```python
from build123d import *

# Parameters (mm, degrees)
SKIZZE1_W                       = 240
SKIZZE1_H                       = 184.5
AUFSATZ_LINEAR_AUSTRAGEN1_DEPTH = 70
SKIZZE2_W                       = 206
SKIZZE2_H                       = 50
SCHNITT_LINEAR_AUSTRAGEN3_DEPTH = 231.955082213
SKIZZE3_W                       = 240
SKIZZE3_H                       = 184.662178294
SKIZZE3_W_2                     = 200
SKIZZE3_H_2                     = 144.5
AUFSATZ_LINEAR_AUSTRAGEN2_DEPTH = 5
F_8_0MM_STIFTLOCH1_D            = 8


with BuildPart() as part:
    # Skizze1 → Aufsatz-Linear austragen1 (new body)
    with BuildSketch(Plane(origin=(0, 0, 0), x_dir=(1, 0, 0), z_dir=(0, 1, 0))):
        Rectangle(SKIZZE1_W, SKIZZE1_H)
        Polygon((103, 87.25), (-103, 87.25), (-103, 75.25), (-115, 75.25), (-115, -75.25), (-103, -75.25), (-103, -87.25), (103, -87.25), (103, -75.25), (115, -75.25), (115, 75.25), (103, 75.25), align=None, mode=Mode.SUBTRACT)
    extrude(amount=AUFSATZ_LINEAR_AUSTRAGEN1_DEPTH)

    # Skizze2 → Schnitt-Linear austragen3 (cut, through all)
    with BuildSketch(Plane.XY.offset(92.25)):
        with Locations((0, 45)):
            Rectangle(SKIZZE2_W, SKIZZE2_H)
    extrude(amount=-SCHNITT_LINEAR_AUSTRAGEN3_DEPTH, mode=Mode.SUBTRACT)

    # Skizze3 → Aufsatz-Linear austragen2 (add)
    with BuildSketch(Plane(origin=(0, 0, 0), x_dir=(1, 0, 0), z_dir=(0, 1, 0))):
        with Locations((0, -0.081089147)):
            Rectangle(SKIZZE3_W, SKIZZE3_H)
        Rectangle(SKIZZE3_W_2, SKIZZE3_H_2, mode=Mode.SUBTRACT)
    extrude(amount=AUFSATZ_LINEAR_AUSTRAGEN2_DEPTH)

    # Skizze7 → Kernloch für M4x0.71 (revolve, cut)
    with BuildSketch(Plane(origin=(107.5, 0, -79.75), x_dir=(0, 0, -1), z_dir=(1, 0, 0))):
        Polygon((0, 0), (0, 20.991420021), (1.65, 20), (1.65, 0), align=None)
    kernloch_f_r_m4x0_71 = revolve(axis=Axis((107.5, -6.35, -79.75), (0, 1, 0)), mode=Mode.SUBTRACT)

    # Spiegeln1: Kernloch für M4x0.71 across plane
    add(kernloch_f_r_m4x0_71.mirror(Plane.ZY), mode=Mode.SUBTRACT)

    # Spiegeln2: Kernloch für M4x0.71 across plane
    add(kernloch_f_r_m4x0_71.mirror(Plane(origin=(0, 0, 0), x_dir=(1, 0, 0), z_dir=(0, 0, -1))), mode=Mode.SUBTRACT)

    # Spiegeln2 copy 1 sketch → Spiegeln2 copy 1 (revolve, cut)
    with BuildSketch(Plane(origin=(-107.5, 0, 79.75), x_dir=(0, 0, 1), z_dir=(-1, 0, 0))):
        Polygon((0, 0), (0, 20.991420021), (1.65, 20), (1.65, 0), align=None)
    revolve(axis=Axis((-107.5, -6.35, 79.75), (0, 1, 0)), mode=Mode.SUBTRACT)

    # Ø8.0mm Stiftloch1 (through all)
    with Locations(Plane.ZY.offset(120)):
        with Locations((-52.25, 55)):
            f_8_0mm_stiftloch1 = Hole(F_8_0MM_STIFTLOCH1_D / 2)

    # Spiegeln3: Ø8.0mm Stiftloch1 across plane
    add(f_8_0mm_stiftloch1.mirror(Plane(origin=(0, 0, 0), x_dir=(1, 0, 0), z_dir=(0, 0, -1))), mode=Mode.SUBTRACT)


solid = part.part
```
Source: CAD feature listing. Evaluate the final solid. Frame: model axes, mm. A direction names the side the tool comes from. Round coordinates to 2 decimals unless told otherwise and drop trailing zeros. Loops run counter-clockwise (first coordinate to the right, second up) from the corner with the lowest first, then second, coordinate; pieces in that order, holes last. Notation, with made-up numbers: M -31,9.25 L 3,9.25 A15 ccw 3,28.25 Z; hole C -12,55.25 d1. An arc over 180 degrees is marked long. Use a Markdown table: item, result. Add a question column.
1. Contact query for flat-ended pins moving along their axis: P1, Ø5.5, axis at x = -5, z = 90.5, coming from the +Y side; P2, Ø1.5, axis at x = -3, y = 20, coming from the +Z side. Output: stop coordinate, or through.
2. Section query B-B on x = -81. Return the cut outline in (y, z), then the cut area to 3 significant figures.
3. Mould query, pull axis X, two halves, no side actions, for faces 6 (the flat face through (100, 2, 1)), 7 (the flat face through (-2, 0, -83)). Classes: pulls with the +X half, pulls with the -X half, needs draft (parallel to the pull), parting line crosses it, or undercut.
4. Section query A-A on z = 38. Return the cut outline in (x, y), then the cut area to 3 significant figures.
5. Section query C-C on z = -52.25. Return the cut outline in (x, y), then the cut area to 3 significant figures.
6. Reachability of faces 1 (the flat face through (109, 37, 75.25)), 2 (the flat face through (-100, 2, 1)), 3 (the flat face through (-2, 2, 92.412)), 4 (the flat face through (-1, 20, -90)), 5 (the cylindrical face through (117.535, 51.095, -51.383)) from +Z, -Z, +X, -X, +Y, -Y: full face, straight path, thin tool, end or side. Return the list, or none.
7. Line query: line 1 (X direction, y = 8, z = 79.75); line 2 (Z direction, x = -107.5, y = 10.75); line 3 (X direction, y = 25, z = 79). Output: solid intervals per line, ascending.
Reported:
| question | item | result |
|---|---|---|
| 1 | P1 | stops at y = 20 |
| 1 | P2 | stops at z = 92.25 |
| 2 | outline | M 0,-92.25 L 20,-92.25 L 20,-87.25 L 5,-87.25 L 5,-72.25 L 0,-72.25 Z; M 0,72.25 L 5,72.25 L 5,87.25 L 20,87.25 L 20,92.25 L 5,92.25 L 5,92.41 L 0,92.41 Z |
| 2 | area | 351 mm² |
| 3 | face 6 | undercut |
| 3 | face 7 | needs draft |
| 4 | outline | M -120,0 L -100,0 L -100,5 L -115,5 L -115,70 L -120,70 Z; M 100,0 L 120,0 L 120,70 L 115,70 L 115,5 L 100,5 Z |
| 4 | area | 850 mm² |
| 5 | outline | M -120,0 L -100,0 L -100,5 L -115,5 L -115,51 L -120,51 Z; M -120,59 L -115,59 L -115,70 L -120,70 Z; M 100,0 L 120,0 L 120,51 L 115,51 L 115,5 L 100,5 Z; M 115,59 L 120,59 L 120,70 L 115,70 Z |
| 5 | area | 770 mm² |
| 6 | face 1 | +Y |
| 6 | face 2 | +Y, -Y |
| 6 | face 3 | +Z, +X, -X, +Y, -Y |
| 6 | face 4 | +Z, -Z, +Y |
| 6 | face 5 | +X, -X |
| 7 | line 1 | x = -120 to -109.15, -105.85 to -103, 103 to 105.85, 109.15 to 120 |
| 7 | line 2 | z = -92.25 to -81.4, -78.1 to -75.25, 75.25 to 78.1, 81.4 to 92.25 |
| 7 | line 3 | x = -120 to -103, 103 to 120 |
